from build123d import *

# Parameters (mm, degrees)
F0_R          = 4
F0_R_2        = 2
F1_DEPTH      = 6
F1_DEPTH_BACK = 6
F2_R          = 2
F3_DEPTH      = 0.5


# Not quite as in the source:
# - a pattern or mirror of a feature is missing from the dataset's text; its kind, count and spacing are read off the source's solid


with BuildPart() as f1:
    # F0 (on Front) → F1 (new body, two sides)
    with BuildSketch(Plane.XZ) as f1_sk:
        Circle(F0_R)
        Circle(F0_R_2, mode=Mode.SUBTRACT)
    extrude(amount=F1_DEPTH)
    extrude(f1_sk.sketch, amount=-F1_DEPTH_BACK)

    # F2 (on face) → F3 (cut)
    with BuildSketch(Plane.XZ.offset(6)):
        with BuildLine():
            Line((1.902670174, 2.902670174), (-1.7521820182, 2.902670174))
            ThreePointArc((-1.7521820182, 2.902670174), (-2.4592887994, 2.6097769551), (-2.7521820182, 1.902670174))
            Line((-2.7521820182, 1.902670174), (-2.7521820182, -1.7521820182))
            ThreePointArc((-2.7521820182, -1.7521820182), (-2.4592887994, -2.4592887994), (-1.7521820182, -2.7521820182))
            Line((-1.7521820182, -2.7521820182), (1.902670174, -2.7521820182))
            ThreePointArc((1.902670174, -2.7521820182), (2.6097769551, -2.4592887994), (2.902670174, -1.7521820182))
            Line((2.902670174, -1.7521820182), (2.902670174, 1.902670174))
            ThreePointArc((2.902670174, 1.902670174), (2.6097769551, 2.6097769551), (1.902670174, 2.902670174))
        make_face()
        Circle(F2_R, mode=Mode.SUBTRACT)
    f3 = extrude(amount=-F3_DEPTH, mode=Mode.SUBTRACT)

    # F3_copies: F3 across plane
    add(f3.mirror(Plane.ZX), mode=Mode.SUBTRACT)


solid = f1.part
Could you check a few things on this model? Use its own coordinates, in mm. A direction names the side the tool comes from. Give positions to 0.01 mm unless a question says otherwise; leave off trailing zeros. Order: outer loops, then holes, each group sorted by start corner. A loop starts at its lowest first (then second) coordinate and runs counter-clockwise, first axis right, second up.
Item 1: If we section it at A-A, the plane z = 0: Write out the boundary of the cut face in (x, y), plus the area to 3 significant figures.
Item 2: If we section it at B-B, the plane x = 0: Write out the boundary of the cut face in (y, z), plus the area to 3 significant figures.
Item 3: For faces 5 (the face through (-2.47, 5.75, -2.45)), 6 (the face through (-3, -6, 0)), 7 (the face through (2.62, -5.75, 2.6)), which set-ups out of +Z, -Z, +X, -X, +Y, -Y let a thin tool reach every point of the face, with its end or its side?
Item 4: I need wall thicknesses on line 1 (Z direction, x = 0, y = -0.5); line 2 (Y direction, x = -1.5, z = -2); line 3 (Z direction, x = -1.5, y = -3.5). Which ranges of each line are inside material? Lowest first, please.
Item 5: I'm going to push flat-ended pins straight in: pin 1 (1 mm diameter, centred on x = -2.5, y = -1, fed in from -Z); pin 2 (0.6 mm diameter, centred on x = 1, y = -5.5, fed in from +Z); pin 3 (1.5 mm diameter, centred on y = 1, z = 1, fed in from -X). Where does each tip first touch, or does it pass through?
Item 6: If we mould it in two halves opening along Z, with no side actions, what happens to faces 1 (the face through (2.62, 5.75, 2.6)), 2 (the face through (-3, 6, 0)), 3 (the face through (-0.867, -0.084, -3.905)), 4 (the face through (2, 5.5, 1))? For each: pulls with the +Z half, pulls with the -Z half, needs draft (parallel to the pull), parting line crosses it, or undercut.
Item 7: If we section it at C-C, the plane y = 3: Write out the boundary of the cut face in (x, z), plus the area to 3 significant figures.
Values:
1. outline: (-4, -6) - (-2.75, -6) - (-2.75, -5.5) - (-2, -5.5) - (-2, 5.5) - (-2.75, 5.5) - (-2.75, 6) - (-4, 6) - close; (2, -5.5) - (2.9, -5.5) - (2.9, -6) - (4, -6) - (4, 6) - (2.9, 6) - (2.9, 5.5) - (2, 5.5) - close
1. area: 46.3 mm2
2. outline: (-6, -4) - (6, -4) - (6, -2.75) - (5.5, -2.75) - (5.5, -2) - (-5.5, -2) - (-5.5, -2.75) - (-6, -2.75) - close; (-6, 2.9) - (-5.5, 2.9) - (-5.5, 2) - (5.5, 2) - (5.5, 2.9) - (6, 2.9) - (6, 4) - (-6, 4) - close
2. area: 46.3 mm2
3. face 5: +Y
3. face 6: +Z, -Z, +X, -X, -Y
3. face 7: -Y
4. line 1: z = -4 to -2, 2 to 4
4. line 2: y = -5.5 to 5.5
4. line 3: z = -3.71 to -1.32, 1.32 to 3.71
5. pin 1: stops at z = -3.46
5. pin 2: stops at z = 3.94
5. pin 3: stops at x = -3.99
6. face 1: undercut
6. face 2: needs draft
6. face 3: parting line crosses it
6. face 4: undercut
7. outline: circle Ø8 at (0, 0); hole circle Ø4 at (0, 0)
7. area: 37.7 mm2
